Check sheet for the modelled part. Datum: model origin and axes. Units: mm. A direction names the side the tool comes from. Round coordinates to 2 decimals unless told otherwise and drop trailing zeros. Loops run counter-clockwise (first coordinate to the right, second up) from the corner with the lowest first, then second, coordinate; pieces in that order, holes last. Notation, with made-up numbers: (-27, 54.25) - (-22, 54.25) arc R10 ccw to (-22, 63.25) - close; hole circle Ø2 at (77, 69.5). An arc over 180 degrees is marked (long way). Put each result on its own line as item: value. Start each with the question number.
Item 1: Tool access check on faces 5 (the flat face through (-264, 408.904, 2057)), 6 (the flat face through (-550.293, 222, 2057)). Record the directions out of +Z, -Z, +X, -X, +Y, -Y that give a thin tool (end or side, any length) a straight path to the whole face; none if there is none.
Item 2: Section check C-C, the plane z = 2034.5. Record the cut outline in (x, y), and give its area (3 significant figures).
Item 3: Section check B-B, the plane y = 248.5. Record the cut outline in (x, z), and give its area (3 significant figures).
Item 4: Material ranges on line 1 along X through (y, z) = (335.5, 2012.5); line 2 along Y through (x, z) = (-10.5, 2060.5), recorded low to high.
Item 5: Section check A-A, the plane x = -29. Record the cut outline in (y, z).
Item 6: Draft check along X on faces 1 (the flat face through (-264, 40.504, 2057)), 2 (the flat face through (-560.293, 222, 2057)), 3 (the flat face through (23.407, 222, 2057)), 4 (the flat face through (-264, 50.504, 2059)). Enter one of: pulls with the +X half, pulls with the -X half, needs draft (parallel to the pull), parting line crosses it, or undercut.
from build123d import *

# Parameters (mm, degrees)
EXTRUDE_START         = -100
EXTRUDE_1_OUTLINE_W   = 579.7
EXTRUDE_1_OUTLINE_H   = 368.4
EXTRUDE_1_OUTLINE_W_2 = 559.7
EXTRUDE_1_OUTLINE_H_2 = 348.4
EXTRUDE_1_DEPTH       = 100
SKETCH_3_W            = 2
SKETCH_3_H            = 368.4
EXTRUDE_2_DEPTH       = 100
SKETCH_4_W            = 2
SKETCH_4_H            = 348.4
CUT_EXTRUDE_3_DEPTH   = 100


# Read off the part's stored shape, not the designer's step: 填料-伸長1
with BuildPart() as part:
    # 填料-伸長1 outline → 填料-伸長1 (new body)
    with BuildSketch(Plane(origin=(0, 0, 2008.045378916), x_dir=(-1, 0, 0), z_dir=(0, 0, -1)).offset(EXTRUDE_START)):
        with Locations((268.443182196, 224.704175019)):
            Rectangle(EXTRUDE_1_OUTLINE_W, EXTRUDE_1_OUTLINE_H)
        with Locations((268.443182196, 224.704175019)):
            Rectangle(EXTRUDE_1_OUTLINE_W_2, EXTRUDE_1_OUTLINE_H_2, mode=Mode.SUBTRACT)
    extrude(amount=EXTRUDE_1_DEPTH)

    # 草圖3 → 填料-伸長2 (add)
    with BuildSketch(Plane(origin=(0, 0, 2008.045378916), x_dir=(-1, 0, 0), z_dir=(0, 0, -1))):
        with Locations((-22.406817804, 224.704175019)):
            Rectangle(SKETCH_3_W, SKETCH_3_H)
        with Locations((559.293182196, 224.704175019)):
            Rectangle(SKETCH_3_W, SKETCH_3_H)
    extrude(amount=-EXTRUDE_2_DEPTH)

    # 草圖4 → 除料-伸長3 (cut)
    with BuildSketch(Plane(origin=(0, 0, 2008.045378916), x_dir=(-1, 0, 0), z_dir=(0, 0, -1))):
        with Locations((-12.406817804, 224.704175019)):
            Rectangle(SKETCH_4_W, SKETCH_4_H)
        with Locations((549.293182196, 224.704175019)):
            Rectangle(SKETCH_4_W, SKETCH_4_H)
    extrude(amount=-CUT_EXTRUDE_3_DEPTH, mode=Mode.SUBTRACT)


solid = part.part
Check result:
1. face 5: +Z, -Z, +X, -X, +Y
1. face 6: +Z, -Z
2. outline: (-560.29, 40.5) - (23.41, 40.5) - (23.41, 408.9) - (-560.29, 408.9) - close; hole (-550.29, 50.5) - (13.41, 50.5) - (13.41, 398.9) - (-550.29, 398.9) - close
2. area: 18,600 mm²
3. outline: (-560.29, 2008.05) - (-550.29, 2008.05) - (-550.29, 2108.05) - (-560.29, 2108.05) - close; (13.41, 2008.05) - (23.41, 2008.05) - (23.41, 2108.05) - (13.41, 2108.05) - close
3. area: 2,000 mm²
4. line 1: -560.29 to -550.29, 13.41 to 23.41
4. line 2: 40.5 to 50.5, 398.9 to 408.9
5. outline: (40.5, 2008.05) - (50.5, 2008.05) - (50.5, 2108.05) - (40.5, 2108.05) - close; (398.9, 2008.05) - (408.9, 2008.05) - (408.9, 2108.05) - (398.9, 2108.05) - close
6. face 1: needs draft
6. face 2: pulls with the -X half
6. face 3: pulls with the +X half
6. face 4: undercut
